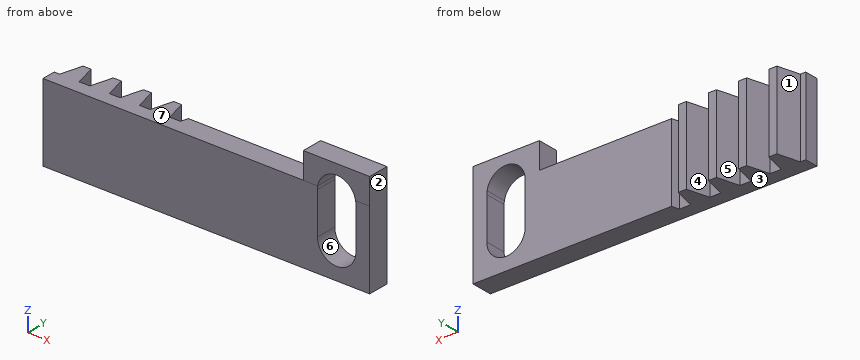
from build123d import *

# Parameters (mm, degrees)
BLANKSKE_W          = 20
BLANKSKE_H          = 5.5
BLANK_DEPTH         = 12
TOOTHCUTSIM_DEPTH   = 24.963513933
TEETHCUTS_COUNT     = 5
TEETHCUTS_PITCH     = 4.712388975
SKETCH2_W           = 12
SKETCH2_H           = 3.278265845
BOSS_EXTRUDE1_DEPTH = 31
CUT_EXTRUDE2_REACH  = 54.495
BOSS_EXTRUDE2_DEPTH = 3.278266
CUT_EXTRUDE3_DEPTH  = 22.5


with BuildPart() as part:
    # BlankSke → Blank (new body)
    with BuildSketch(Plane.XY):
        with Locations((10, 2.75)):
            Rectangle(BLANKSKE_W, BLANKSKE_H)
    extrude(amount=-BLANK_DEPTH)

    # TooCutSkeSim → ToothCutSim (cut, through all)
    with BuildSketch(Plane.XY):
        Polygon((0.852189273, 2.125), (-0.852189273, 2.125), (-1.731592507, 5.5254), (1.731592507, 5.5254), align=None)
    toothcutsim = extrude(amount=-TOOTHCUTSIM_DEPTH, mode=Mode.SUBTRACT)

    # TeethCuts: ToothCutSim ×5
    with Locations(*[(i * TEETHCUTS_PITCH, 0, 0) for i in range(1, TEETHCUTS_COUNT)]):
        add(toothcutsim, mode=Mode.SUBTRACT)

    # Sketch2 → Boss-Extrude1 (add)
    with BuildSketch(Plane(origin=(20, 0, 0), x_dir=(0, 0, -1), z_dir=(1, 0, 0))):
        with Locations((6, 1.639132923)):
            Rectangle(SKETCH2_W, SKETCH2_H)
    extrude(amount=BOSS_EXTRUDE1_DEPTH)

    # Sketch3 → Cut-Extrude2 (cut, up to next)
    with BuildSketch(Plane(origin=(0, 3.278265845, 0), x_dir=(1, 0, 0), z_dir=(0, 1, 0)), mode=Mode.PRIVATE) as cut_extrude2_sk1:
        with BuildLine():
            Line((48.847, 7), (48.847, 5))
            ThreePointArc((48.847, 5), (45.847, 2), (42.847, 5))
            Line((42.847, 5), (42.847, 7))
            ThreePointArc((42.847, 7), (45.847, 10), (48.847, 7))
        make_face()
    cut_extrude2_tool1 = extrude(cut_extrude2_sk1.sketch, amount=-CUT_EXTRUDE2_REACH, mode=Mode.PRIVATE) & part.part
    add(cut_extrude2_tool1.solids().sort_by_distance((45.847, 3.278266, -6))[0], mode=Mode.SUBTRACT)

    # Sketch5 → Boss-Extrude2 (add)
    with BuildSketch(Plane(origin=(0, 3.278265845, 0), x_dir=(1, 0, 0), z_dir=(0, 1, 0))):
        with BuildLine():
            Line((42.890323487, 0), (40.636775161, 0))
            Line((40.636775161, 0), (40.636775161, -4.064))
            Line((40.636775161, -4.064), (51, -4.064))
            Line((51, -4.064), (51, 0))
            Line((51, 0), (48.803676513, 0))
            ThreePointArc((48.803676513, 0), (45.847, -2.492), (42.890323487, 0))
        make_face()
    extrude(amount=-BOSS_EXTRUDE2_DEPTH)

    # Sketch6 → Cut-Extrude3 (cut)
    with BuildSketch(Plane(origin=(0, 3.278265845, 0), x_dir=(1, 0, 0), z_dir=(0, 1, 0))):
        with BuildLine():
            Line((48.847, 7), (48.847, 0.508))
            ThreePointArc((48.847, 0.508), (45.847, -2.492), (42.847, 0.508))
            Line((42.847, 0.508), (42.847, 7))
            ThreePointArc((42.847, 7), (45.847, 10), (48.847, 7))
        make_face()
    extrude(amount=-CUT_EXTRUDE3_DEPTH, mode=Mode.SUBTRACT)


solid = part.part
Read the model definition and answer for the solid it produces. Units are mm, in the model's axes. Face numbers are marked on the shaded views. A direction names the side the tool comes from. Coordinates: 2 decimals unless noted, no trailing zeros. Write each loop counter-clockwise with the first axis right and the second up, starting at its lowest first coordinate (ties: lowest second). Pieces come first, ordered by that corner, then holes. Notation, with made-up numbers: (-15.5, 23.5) -> (20.5, 23.5) arc R25 cw to (20.5, 62.5) -> close; hole circle Ø4 at (18.5, 75). An arc over 180 degrees is marked (long way). Return JSON: item names as keys, results as strings.
(1) The part is cut by section C-C on x = 28. Give the vertices of the cut face in (y, z), then the cut area to 3 significant figures.
Answers below:
{"outline": "(0, -12) -> (3.28, -12) -> (3.28, 0) -> (0, 0) -> close", "area": "39.3 mm^2"}
(2) The part is cut by section B-B on z = -9. Give the vertices of the cut face in (x, y) (3 decimals).
Answers below:
{"outline": "(0, 0) -> (43.611, 0) -> (43.611, 3.278) -> (20, 3.278) -> (19.702, 2.125) -> (17.997, 2.125) -> (17.125, 5.5) -> (15.862, 5.5) -> (14.989, 2.125) -> (13.285, 2.125) -> (12.412, 5.5) -> (11.15, 5.5) -> (10.277, 2.125) -> (8.573, 2.125) -> (7.7, 5.5) -> (6.437, 5.5) -> (5.565, 2.125) -> (3.86, 2.125) -> (2.987, 5.5) -> (1.725, 5.5) -> (0.852, 2.125) -> (0, 2.125) -> close; (48.083, 0) -> (51, 0) -> (51, 3.278) -> (48.083, 3.278) -> close"}
(3) For a pull along X with two mould halves and no side action, classify the marked faces 1, 2, 3 and 4 as pulls with the +X half, pulls with the -X half, needs draft (parallel to the pull), parting line crosses it, or undercut.
Answers below:
{"face 1": "pulls with the -X half", "face 2": "pulls with the +X half", "face 3": "needs draft", "face 4": "undercut"}
(4) Each of these flat-tipped pins is pushed along its axis until it touches: P1, Ø1.4, axis at x = 9.5, z = -5.5, coming from the +Y side (3 decimals); P2, Ø6, axis at x = 30.5, z = -3.5, coming from the +Y side; P3, Ø1, axis at y = 1.5, z = 2.5, coming from the -X side; P4, Ø3, axis at y = 5, z = 2, coming from the +X side. Where does it stop, or does it pass through?
Answers below:
{"P1": "y = 2.125", "P2": "y = 3.28", "P3": "x = 40.64", "P4": "through"}
(5) Which of the six approach directions +Z, -Z, +X, -X, +Y, -Y give full straight-line access (tool end or side, diameter ignored) to the marked faces 5, 6 and 7?
Answers below:
{"face 5": "+Z, -Z, +Y", "face 6": "+Y, -Y", "face 7": "+Z, -X, +Y, -Y"}
(6) The part is cut by section A-A on y = 1.5. Give the vertices of the cut face in (x, z), then the cut area to 3 significant figures.
Answers below:
{"outline": "(0, -12) -> (51, -12) -> (51, 4.06) -> (40.64, 4.06) -> (40.64, 0) -> (0, 0) -> close; hole (42.85, -7) arc R3 ccw to (48.85, -7) -> (48.85, -0.51) arc R3 ccw to (42.85, -0.51) -> close", "area": "587 mm^2"}
(7) Consider line 1 along X through (y, z) = (4.6, -0.5); line 2 along X through (y, z) = (1.3, -7); line 3 along X through (y, z) = (4.85, -7.25). Determine where each line is inside the solid, lowest interval first. Write a range as from..to.
Answers below:
{"line 1": "1.49..3.22, 6.2..7.93, 10.92..12.64, 15.63..17.36", "line 2": "0..42.85, 48.85..51", "line 3": "1.56..3.16, 6.27..7.87, 10.98..12.58, 15.69..17.29"}
